The model under review builds one solid part; all positions refer to its coordinate system, in mm. A direction names the side the tool comes from. Coordinates: 2 decimals unless noted, no trailing zeros. Loops run counter-clockwise (first coordinate to the right, second up) from the corner with the lowest first, then second, coordinate; pieces in that order, holes last. Notation, with made-up numbers: M 2.5,66 L 46.5,66 A16 cw 46.5,72 Z; hole C -32,50 d6. An arc over 180 degrees is marked long. Use CSV: the item, a comma, the result in double quotes. Start each with the question number.
1. Draft analysis for pull direction Z (two halves, no side actions). For faces 3 (the flat face through (-9, -7, 6)), 4 (the cylindrical face through (-19.21, -21.28, 3.65)), 5 (the cylindrical face through (-7.542, -21.407, 2.697)), 6 (the cylindrical face through (-14.84, -11.7, 15.86)), state which applies: +Z half, -Z half, draft (parallel to the pull), parting line (faces both ways), or undercut.
2. Tool access review of faces 1 (the flat face through (-10.5, -20, 13)), 2 (the flat face through (-9, -20, 0)): name each direction out of +Z, -Z, +X, -X, +Y, -Y from which nothing blocks a thin tool from reaching the whole face with its end or side.
3. Clearance check with flat-ended pins moving along their axes: P1, Ø10, axis at x = -15, z = 15, coming from the +Y side; P2, Ø2, axis at y = -20.04, z = 3, coming from the +X side; P3, Ø3, axis at x = -10, z = 19, coming from the -Y side; P4, Ø5, axis at x = -19, z = 11, coming from the +Y side. State where each tip first meets the part, or that it passes through.
4. Add section D-D, the plane y = -31. Write out the cut boundary in (x, z).
5. Add section A-A, the plane y = -41. Write out the cut boundary in (x, z).
6. Add section C-C, the plane x = -19. Write out the cut boundary in (y, z), then the cut area to 3 significant figures.
7. For L1, parallel to X at y = -3.5, z = 3.95; L2, parallel to Y at x = -9.5, z = 1.5; L3, parallel to Y at x = -13, z = 2.8, list the stretches that pass through material, from the lowest coordinate up.
8. Add section B-B, the plane z = 2.75. Write out the cut boundary in (x, y), then the cut area to 3 significant figures.
Autodesk Inventor part; units mm, degrees
ref_plane "YZ Plane" through (0, 0, 0) normal (1, 0, 0) x (0, 1, 0)
ref_plane "XZ Plane" through (0, 0, 0) normal (0, 1, 0) x (-1, 0, 0)
ref_plane "XY Plane" through (0, 0, 0) normal (0, 0, 1) x (1, 0, 0)
ref_plane "Arbeitsebene1" through (0, 0, 0) normal (0, 0, 1) x (1, 0, 0)
sketch "Skizze1" plane through (0, 0, 0) normal (0, 0, 1) x (1, 0, 0)
  circle A0 centre (-13, -20) radius 11
  circle A1 centre (-13, -36.5) radius 2
  circle A2 centre (-13, -3.5) radius 2
  line L0 (0, 0) -> (0, -9.8388)
  line L1 (-29, 0) -> (0, 0)
  line L2 (-33, -4) -> (-29, 0)
  line L3 (-33, -4) -> (-33, -36)
  line L4 (-29, -40) -> (-33, -36)
  line L5 (0, -40) -> (-29, -40)
  line L6 (0, -30.1612) -> (0, -40)
  arc A3 (0, -30.1612) -> (0, -9.8388) centre (-13, -20) ccw
  circle A4 centre (-13, -3.5) radius 5
  circle A5 centre (-13, -36.5) radius 5
  circle A6 centre (-13, -20) radius 2.5
  line L7 (-13, -3.5) -> (-13, -36.5) construction
  line L8 (-21.5, -3.5) -> (-21.5, -36.5)
  line L9 (-4.5, -36.5) -> (-4.5, -3.5)
  arc A7 (-4.5, -3.5) -> (-21.5, -3.5) centre (-13, -3.5) ccw
  arc A8 (-21.5, -36.5) -> (-4.5, -36.5) centre (-13, -36.5) ccw
  line L10 (-18, -20) -> (-10.5, -15.6699)
  line L11 (-10.5, -15.6699) -> (-10.5, -24.3301)
  line L12 (-10.5, -24.3301) -> (-18, -20)
  point P0 (-13, -20)
  point P1 (-13, -20)
  dimension "d0" = 10
  dimension "d1" = 10
  dimension "d2" = 5
  dimension "d3" = 17
extrude "Extrusion1" add sketch "Skizze1" along normal blind 6 contours L9 A0 L8 | A0 L8 A7 L1 A4 L9 | L9 A8 L5 A5 L8 A0 | L1 A4 A7 | A8 L5 A5
sketch "Skizze2" plane through (-21.5, -36.5, 0) normal (-1, 0, 0) x (0, 0, 1)
  line L0 (6, 19) -> (0, 19)
  line L1 (6, 14) -> (0, 14)
  circle A0 centre (3, 16.4602) radius 1.4
  point P0 (0, 36.5)
  dimension "d6" = 2.8
extrude "Extrusion2" cut sketch "Skizze2" against normal through all
sketch "Skizze3" plane through (0, 0, 6) normal (0, 0, 1) x (1, 0, 0)
  point P0 (0, 0)
sketch "Skizze4" plane through (0, 0, 6) normal (0, 0, 1) x (1, 0, 0)
  line L0 (-21.5, -3.5) -> (-21.5, -36.5)
  arc A0 (-21.5, -36.5) -> (-4.5, -36.5) centre (-13, -36.5) ccw
  line L1 (-4.5, -36.5) -> (-4.5, -3.5)
  arc A1 (-4.5, -3.5) -> (-21.5, -3.5) centre (-13, -3.5) ccw
  circle A2 centre (-13, -36.5) radius 5
  circle A3 centre (-13, -3.5) radius 5
  line L2 (-18, -20) -> (-10.5, -15.6699)
  line L3 (-10.5, -15.6699) -> (-10.5, -24.3301)
  line L4 (-10.5, -24.3301) -> (-18, -20)
  circle A4 centre (-13, -20) radius 2.5
  circle A5 centre (-13, -20) radius 8.5
  point P0 (0, 0)
  dimension "d9" = 5
extrude "Extrusion3" add sketch "Skizze4" along normal blind 20 contours A5
properties part number "40_XYZstage_micrometer_motorized_nema8_samplemount_lightsheet_feptube50_screwed"
Computed:
1,face 3,"+Z half"
1,face 4,"undercut"
1,face 5,"undercut"
1,face 6,"draft"
2,face 1,"+Z, -Z"
2,face 2,"-Z, +X, -X, +Y, -Y"
3,P1,"stops at y = -11.5"
3,P2,"passes through"
3,P3,"stops at y = -28.37"
3,P4,"stops at y = -12.25"
4,outline,"M -21.5,0 L -4.5,0 L -4.5,6 L -21.5,6 Z"
5,outline,"M -20.21,0 L -15.18,0 L -15.18,6 L -20.21,6 Z; M -10.82,0 L -5.79,0 L -5.79,6 L -10.82,6 Z"
6,outline,"M -42.52,0 L 2.52,0 L 2.52,6 L -13.98,6 L -13.98,26 L -26.02,26 L -26.02,6 L -42.52,6 Z; hole C -20.04,3 d2.8"
6,area,"505 mm^2"
7,L1,"x = -21.5 to -18, -8 to -4.5"
7,L2,"y = -44.25 to -40.07, -32.93 to -7.07, 0.07 to 4.25"
7,L3,"y = -45 to -41.5, -31.5 to -22.89, -17.11 to -8.5, 1.5 to 5"
8,outline,"M -21.5,-36.5 A8.5 ccw -4.5,-36.5 L -4.5,-21.42 L -10.5,-21.42 L -10.5,-24.33 L -15.55,-21.42 L -21.5,-21.42 Z; M -21.5,-18.66 L -15.68,-18.66 L -10.5,-15.67 L -10.5,-18.66 L -4.5,-18.66 L -4.5,-3.5 A8.5 ccw -21.5,-3.5 Z; hole C -13,-36.5 d10; hole C -13,-3.5 d10"
8,area,"569 mm^2"
